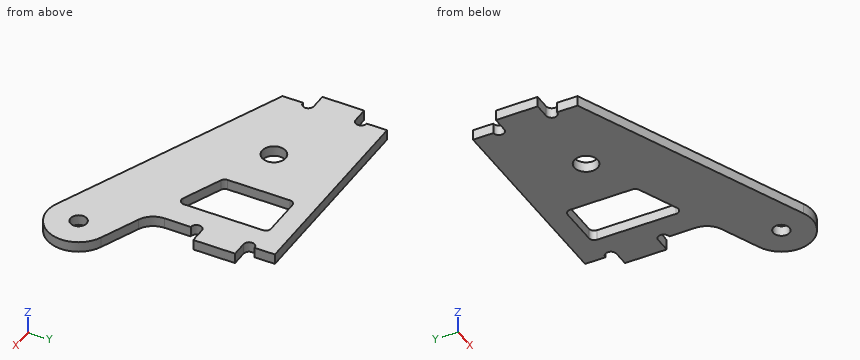
Autodesk Inventor part; units mm, degrees
ref_plane "YZ Plane" through (0, 0, 0) normal (1, 0, 0) x (0, 1, 0)
ref_plane "XZ Plane" through (0, 0, 0) normal (0, 1, 0) x (-1, 0, 0)
ref_plane "XY Plane" through (0, 0, 0) normal (0, 0, 1) x (1, 0, 0)
sketch "スケッチ1" plane through (0, 0, 0) normal (0, 0, 1) x (1, 0, 0)
  line L0 (-19.75, 25.75) -> (19.75, 25.75) construction
  line L1 (19.75, 25.75) -> (19.75, -25.75) construction
  line L2 (19.75, -25.75) -> (-19.75, -25.75) construction
  line L3 (-19.75, -25.75) -> (-19.75, 25.75) construction
  line L4 (-19.75, 25.75) -> (19.75, -25.75) construction
  line L5 (19.75, 25.75) -> (-19.75, -25.75) construction
  circle A0 centre (27.25, -24.25) radius 1.55
  circle A1 centre (-4.75, -4.25) radius 2.25
  line L6 (0, 25.75) -> (0, -25.75) construction
  line L7 (-19.75, 3.25) -> (-22.75, 3.25)
  line L8 (-22.75, 3.25) -> (-22.75, -4.75)
  arc A2 (-19.75, 3.25) -> (-19.75, 5.35) centre (-19.75, 4.3) ccw
  line L9 (-22.75, -0.75) -> (-19.75, -0.75) construction
  line L10 (-19.75, -4.75) -> (-22.75, -4.75)
  arc A3 (-19.75, -6.85) -> (-19.75, -4.75) centre (-19.75, -5.8) ccw
  line L11 (-19.75, 5.35) -> (-19.75, 9.25)
  line L12 (-19.75, 9.25) -> (19.75, 9.25)
  line L13 (22.75, 3.25) -> (22.75, -4.75)
  arc A4 (19.75, 5.35) -> (19.75, 3.25) centre (19.75, 4.3) ccw
  line L14 (19.75, -4.75) -> (22.75, -4.75)
  arc A5 (19.75, -4.75) -> (19.75, -6.85) centre (19.75, -5.8) ccw
  line L15 (19.75, 5.35) -> (19.75, 9.25)
  line L16 (19.75, 3.25) -> (22.75, 3.25)
  arc A6 (24.8985, -29.77) -> (29.6015, -18.73) centre (27.25, -24.25) ccw
  line L17 (-19.75, -6.85) -> (-19.75, -10.75)
  line L18 (-19.75, -10.75) -> (24.8985, -29.77)
  line L19 (19.75, -6.85) -> (19.75, -14.5333)
  line L20 (19.75, -14.5333) -> (29.6015, -18.73)
  circle A7 centre (-4.75, -4.25) radius 6 construction
  circle A8 centre (27.25, -24.25) radius 6 construction
  line L21 (5.25, 5.25) -> (14.75, 5.25)
  line L22 (14.75, 5.25) -> (14.75, -12.4033)
  line L23 (14.75, -12.4033) -> (5.25, -8.3564)
  line L24 (5.25, -8.3564) -> (5.25, 5.25)
  point P0 (0, 0)
  dimension "d0" = 39.5
  dimension "d1" = 51.5
  dimension "d2" = 3.1
  dimension "d3" = 4.5
  dimension "d4" = 32
  dimension "d5" = 20
  dimension "d6" = 3
  dimension "d7" = 1.05
  dimension "d8" = 8
  dimension "d9" = 26.5
  dimension "d11" = 30
  dimension "d12" = 15
  dimension "d13" = 6
  dimension "d14" = 12
  dimension "d19" = 12
  dimension "d20" = 12
  dimension "d21" = 4
  dimension "d22" = 5
  dimension "d24" = 4
extrude "押し出し1" add sketch "スケッチ1" along normal blind 2
fillet "フィレット1" radius 4 1 edges at (19.75, -14.5333, 1)
fillet "フィレット2" radius 1 4 edges at (5.25, 5.25, 1) (14.75, 5.25, 1) (5.25, -8.3564, 1) (14.75, -12.4033, 1)
equation "\"d24\" = d21"
properties part number "Leg_Joint_side_frame" material "アルミニウム 2014-T4"
The model under review builds one solid part; all positions refer to its coordinate system, in mm. Give positions to 0.01 mm unless a question says otherwise; leave off trailing zeros. Write each loop counter-clockwise with the first axis right and the second up, starting at its lowest first coordinate (ties: lowest second). Pieces come first, ordered by that corner, then holes. Notation, with made-up numbers: (-31.75, -13.75) -> (-14.75, -13.75) arc R30 ccw to (-14.75, 18.25) -> close; hole circle Ø11 at (-31, 31.5). An arc over 180 degrees is marked (long way). Answer in a Markdown table with one row per item.
1) Add section B-B on y = -24.25. State the section outline as (x, z) points, plus the area to 3 significant figures.
Worked answers:
| item | result |
|---|---|
| outline | (11.94, 0) -> (25.7, 0) -> (25.7, 2) -> (11.94, 2) -> close; (28.8, 0) -> (33.25, 0) -> (33.25, 2) -> (28.8, 2) -> close |
| area | 36.4 mm² |
2) Add section D-D on y = 7.5. State the section outline as (x, z) points, plus the area to 3 significant figures.
Worked answers:
| item | result |
|---|---|
| outline | (-19.75, 0) -> (19.75, 0) -> (19.75, 2) -> (-19.75, 2) -> close |
| area | 79.0 mm² |
3) For L1, parallel to X at y = -1, z = 1.1; L2, parallel to X at y = -5.5, z = 1.75; L3, parallel to X at y = -9.5, z = 0.65, list the stretches that pass through material, from the lowest coordinate up. Write a range as [from, to].
Worked answers:
| item | result |
|---|---|
| L1 | [-22.75, 5.25], [14.75, 22.75] |
| L2 | [-18.74, -6.62], [-2.88, 5.25], [14.75, 18.74] |
| L3 | [-19.75, 7.93], [14.75, 19.75] |
4) Add section A-A on z = 1.5. Count the separate pieces of the cut face and the enclosed holes in it, plus the area to 3 significant figures.
Worked answers:
| item | result |
|---|---|
| separate pieces | 1 |
| enclosed holes | 3 |
| area | 1,150 mm² |
5) Clearance check with flat-ended pins moving along their axes: P1, Ø4, axis at x = -2, y = -1.5, coming from the -Z side; P2, Ø1, axis at x = 23, z = 1, coming from the -Y side; P3, Ø0.6, axis at y = -9, z = 1, coming from the -X side; P4, Ø0.6, axis at x = -21, z = 1.5, coming from the -Y side. State where each tip first meets the part, or that it passes through.
Worked answers:
| item | result |
|---|---|
| P1 | z = 0 |
| P2 | y = -29.17 |
| P3 | x = -19.75 |
| P4 | y = -4.75 |
6) Add section C-C on x = 9.5. State the section outline as (y, z) points, plus the area to 3 significant figures.
Worked answers:
| item | result |
|---|---|
| outline | (-23.21, 0) -> (-10.17, 0) -> (-10.17, 2) -> (-23.21, 2) -> close; (5.25, 0) -> (9.25, 0) -> (9.25, 2) -> (5.25, 2) -> close |
| area | 34.1 mm² |
